Verification items for the finished model (mm, model axes). A direction names the side the tool comes from. Coordinates: 2 decimals unless noted, no trailing zeros. Order: outer loops, then holes, each group sorted by start corner. A loop starts at its lowest first (then second) coordinate and runs counter-clockwise, first axis right, second up. Notation, with made-up numbers: M -13.5,79.25 L 0.5,79.25 A24 ccw 0.5,91.25 Z; hole C 63,69 d6. An arc over 180 degrees is marked long. Return JSON: item names as keys, results as strings.
```python
from build123d import *

# Parameters (mm, degrees)
SKETCH2_W           = 100
SKETCH2_H           = 40
BOSS_EXTRUDE5_DEPTH = 14
SHELL1_T            = -2
SKETCH3_6_R         = 2.5
SKETCH3_6_R_2       = 1.5
CUT_EXTRUDE8_DEPTH  = 56.641710973
CUT_EXTRUDE9_DEPTH  = 12
SKETCH5_W           = 100
SKETCH5_H           = 14
SKETCH5_W_2         = 96
SKETCH5_H_2         = 10
BOSS_EXTRUDE6_DEPTH = 5
SKETCH6_R           = 3
SKETCH6_R_2         = 1.5
SKETCH6_R_3         = 1.58
SKETCH6_R_4         = 1.95
BOSS_EXTRUDE7_DEPTH = 14
SKETCH6_2_R         = 1.5
CUT_EXTRUDE11_DEPTH = 58.628118137
CUT_EXTRUDE12_START = -2
SKETCH6_3_R         = 1.58
SKETCH6_3_R_2       = 1.95
CUT_EXTRUDE12_DEPTH = 56.628118137


with BuildPart() as part:
    # Sketch2 → Boss-Extrude5 (new body)
    with BuildSketch(Plane(origin=(0, 0, 0), x_dir=(1, 0, 0), z_dir=(0, 1, 0))):
        Rectangle(SKETCH2_W, SKETCH2_H)
    extrude(amount=BOSS_EXTRUDE5_DEPTH)

    # Shell1
    shell1_openings = [part.faces().sort_by_distance(p)[0] for p in [
        (0, 7, -20),
        (0, 7, 20),
    ]]
    offset(amount=SHELL1_T, openings=shell1_openings, kind=Kind.INTERSECTION)

    # Sketch3<6> → Cut-Extrude8 (cut, through all)
    with BuildSketch(Plane(origin=(0, 14, 0), x_dir=(1, 0, 0), z_dir=(0, 1, 0))):
        with Locations(Location((-10.944299399, 10.466797681, 0), (0, 0, 270))):
            Circle(SKETCH3_6_R)
        with Locations(Location((-42.214291858, -10, 0), (0, 0, 270))):
            Circle(SKETCH3_6_R_2)
        with Locations(Location((-42.214291858, 10, 0), (0, 0, 270))):
            Circle(SKETCH3_6_R_2)
        with Locations(Location((-22.547984959, 10.466797681, 0), (0, 0, 270))):
            Circle(SKETCH3_6_R_2)
        with Locations(Location((-7.3745, -1.251, 0), (0, 0, 270))):
            Circle(SKETCH3_6_R_2)
        with Locations(Location((7.3745, -1.251, 0), (0, 0, 270))):
            Circle(SKETCH3_6_R_2)
        with Locations(Location((12.650652812, 9.804528549, 0), (0, 0, 270))):
            Circle(SKETCH3_6_R_2)
        with Locations(Location((22.400652812, 9.804528549, 0), (0, 0, 270))):
            Circle(SKETCH3_6_R_2)
        with BuildLine():
            ThreePointArc((7.3745, -15), (14.495799481, -13.012041395), (19.557771218, -7.623040759))
            ThreePointArc((19.557771218, -7.623040759), (18.923772695, -5.598677681), (16.899409617, -6.232676204))
            ThreePointArc((16.899409617, -6.232676204), (12.941948405, -10.445809365), (7.3745, -12))
            ThreePointArc((7.3745, -12), (5.8745, -13.5), (7.3745, -15))
        make_face()
        with BuildLine():
            ThreePointArc((-7.3745, -15), (-14.495799481, -13.012041395), (-19.557771218, -7.623040759))
            ThreePointArc((-19.557771218, -7.623040759), (-18.923772695, -5.598677681), (-16.899409617, -6.232676204))
            ThreePointArc((-16.899409617, -6.232676204), (-12.941948405, -10.445809365), (-7.3745, -12))
            ThreePointArc((-7.3745, -12), (-5.8745, -13.5), (-7.3745, -15))
        make_face()
        with Locations(Location((42.150652812, 10, 0), (0, 0, 270))):
            Circle(SKETCH3_6_R_2)
        with Locations(Location((42.150652812, -10, 0), (0, 0, 270))):
            Circle(SKETCH3_6_R_2)
    extrude(amount=-CUT_EXTRUDE8_DEPTH, mode=Mode.SUBTRACT)

    # Sketch3 → Cut-Extrude9 (cut)
    # profile 1 of 2: a face of its own
    with BuildSketch(Plane(origin=(0, 14, 0), x_dir=(1, 0, 0), z_dir=(0, 1, 0))):
        with BuildLine():
            ThreePointArc((-23.545313619, -9.708587593), (-21.009319529, -1.611135279), (-12.911867215, -4.14712937))
            ThreePointArc((-12.911867215, -4.14712937), (-10.611171791, -6.596461319), (-7.3745, -7.5))
            ThreePointArc((-7.3745, -7.5), (-1.3745, -13.5), (-7.3745, -19.5))
            ThreePointArc((-7.3745, -19.5), (-16.826576095, -16.861389441), (-23.545313619, -9.708587593))
        make_face()
        with BuildLine():
            ThreePointArc((-7.3745, -15), (-14.495799481, -13.012041395), (-19.557771218, -7.623040759))
            ThreePointArc((-19.557771218, -7.623040759), (-18.923772695, -5.598677681), (-16.899409617, -6.232676204))
            ThreePointArc((-16.899409617, -6.232676204), (-12.941948405, -10.445809365), (-7.3745, -12))
            ThreePointArc((-7.3745, -12), (-5.8745, -13.5), (-7.3745, -15))
        make_face(mode=Mode.SUBTRACT)
    # profile 2 of 2: a face of its own
    with BuildSketch(Plane(origin=(0, 14, 0), x_dir=(1, 0, 0), z_dir=(0, 1, 0))):
        with BuildLine():
            ThreePointArc((7.3745, -19.5), (16.826576095, -16.861389441), (23.545313619, -9.708587593))
            ThreePointArc((23.545313619, -9.708587593), (21.009319529, -1.611135279), (12.911867215, -4.14712937))
            ThreePointArc((12.911867215, -4.14712937), (10.611171791, -6.596461319), (7.3745, -7.5))
            ThreePointArc((7.3745, -7.5), (1.3745, -13.5), (7.3745, -19.5))
        make_face()
        with BuildLine():
            ThreePointArc((19.557771218, -7.623040759), (18.923772695, -5.598677681), (16.899409617, -6.232676204))
            ThreePointArc((16.899409617, -6.232676204), (12.941948405, -10.445809365), (7.3745, -12))
            ThreePointArc((7.3745, -12), (5.8745, -13.5), (7.3745, -15))
            ThreePointArc((7.3745, -15), (14.495799481, -13.012041395), (19.557771218, -7.623040759))
        make_face(mode=Mode.SUBTRACT)
    extrude(amount=-CUT_EXTRUDE9_DEPTH, mode=Mode.SUBTRACT)

    # Sketch5 → Boss-Extrude6 (add)
    with BuildSketch(Plane.XY.offset(20)):
        with Locations((0, 7)):
            Rectangle(SKETCH5_W, SKETCH5_H)
        with Locations((0, 7)):
            Rectangle(SKETCH5_W_2, SKETCH5_H_2, mode=Mode.SUBTRACT)
    extrude(amount=BOSS_EXTRUDE6_DEPTH)

    # Sketch6 → Boss-Extrude7 (add, through all)
    # profile 1 of 5: a face of its own
    with BuildSketch(Plane(origin=(0, 14, 0), x_dir=(1, 0, 0), z_dir=(0, 1, 0))):
        with Locations(Location((0, 17, 0), (0, 0, 90))):
            Circle(SKETCH6_R)
        with Locations(Location((0, 17, 0), (0, 0, 270))):
            Circle(SKETCH6_R_2, mode=Mode.SUBTRACT)
    # profile 2 of 5: a face of its own
    with BuildSketch(Plane(origin=(0, 14, 0), x_dir=(1, 0, 0), z_dir=(0, 1, 0))):
        with Locations(Location((0, -22, 0), (0, 0, 270))):
            Circle(SKETCH6_R)
        with Locations(Location((0, -22, 0), (0, 0, 270))):
            Circle(SKETCH6_R_2, mode=Mode.SUBTRACT)
    # profile 3 of 5: a face of its own
    with BuildSketch(Plane(origin=(0, 14, 0), x_dir=(1, 0, 0), z_dir=(0, 1, 0))):
        with Locations(Location((9.804442129, 19.091797681, 0), (0, 0, 144.913560917))):
            Circle(SKETCH6_R_3)
    # profile 4 of 5: a face of its own
    with BuildSketch(Plane(origin=(0, 14, 0), x_dir=(1, 0, 0), z_dir=(0, 1, 0))):
        with Locations(Location((9.804442129, 1.841797681, 0), (0, 0, 270))):
            Circle(SKETCH6_R_3)
    # profile 5 of 5: a face of its own
    with BuildSketch(Plane(origin=(0, 14, 0), x_dir=(1, 0, 0), z_dir=(0, 1, 0))):
        with Locations(Location((-0.944299399, 10.466797681, 0), (0, 0, 270))):
            Circle(SKETCH6_R_4)
    extrude(amount=-BOSS_EXTRUDE7_DEPTH)

    # Sketch6<2> → Cut-Extrude11 (cut, through all)
    with BuildSketch(Plane(origin=(0, 14, 0), x_dir=(1, 0, 0), z_dir=(0, 1, 0))):
        with Locations(Location((0, -22, 0), (0, 0, 270))):
            Circle(SKETCH6_2_R)
        with Locations(Location((0, 17, 0), (0, 0, 270))):
            Circle(SKETCH6_2_R)
    extrude(amount=-CUT_EXTRUDE11_DEPTH, mode=Mode.SUBTRACT)

    # Sketch6<3> → Cut-Extrude12 (cut, through all)
    with BuildSketch(Plane(origin=(0, 14, 0), x_dir=(1, 0, 0), z_dir=(0, 1, 0)).offset(CUT_EXTRUDE12_START)):
        with Locations((9.804442129, 19.091797681)):
            Circle(SKETCH6_3_R)
        with Locations(Location((9.804442129, 1.841797681, 0), (0, 0, 270))):
            Circle(SKETCH6_3_R)
        with Locations(Location((-0.944299399, 10.466797681, 0), (0, 0, 270))):
            Circle(SKETCH6_3_R_2)
    extrude(amount=-CUT_EXTRUDE12_DEPTH, mode=Mode.SUBTRACT)


solid = part.part
```
Q1. Tool access check on faces 1 (the face through (13.012, 1.014, 10.403)), 2 (the face through (0, 7, -14)), 3 (the face through (-48, 7, 2)), 4 (the face through (16.71, 13.01, 16.93)). Record the directions out of +Z, -Z, +X, -X, +Y, -Y that give a thin tool (end or side, any length) a straight path to the whole face; none if there is none.
Values:
{"face 1": "+Y, -Y", "face 2": "none", "face 3": "+Z, -Z", "face 4": "+Y"}
Q2. Cross-section at B-B, the plane y = 4.5. Record the boundary of the cut face in (x, z), and give its area (3 significant figures).
Values:
{"outline": "M -50,-20 L -48,-20 L -48,25 L -50,25 Z; C 0,-17 d6; C 0,22 d6; M 48,-20 L 50,-20 L 50,25 L 48,25 Z; hole C 0,-17 d3; hole C 0,22 d3", "area": "222 mm^2"}
Q3. Cross-section at C-C, the plane z = 13.5. Record the boundary of the cut face in (x, y), and give its area (3 significant figures).
Values:
{"outline": "M -50,0 L -13.62,0 L -13.62,2 L -48,2 L -48,12 L -20.9,12 L -20.9,14 L -50,14 Z; M -5.87,0 L 5.87,0 L 5.87,2 L -5.87,2 Z; M -1.37,12 L 1.37,12 L 1.37,14 L -1.37,14 Z; M 13.62,0 L 50,0 L 50,14 L 20.9,14 L 20.9,12 L 48,12 L 48,2 L 13.62,2 Z", "area": "331 mm^2"}
Q4. Cross-section at D-D, the plane z = -16.5. Record the boundary of the cut face in (x, y).
Values:
{"outline": "M -50,0 L -1.41,0 L -1.41,14 L -50,14 Z; M 1.41,0 L 50,0 L 50,14 L 1.41,14 Z; hole M -48,2 L -2.96,2 L -2.96,12 L -48,12 Z; hole M 2.96,2 L 48,2 L 48,12 L 2.96,12 Z"}
Q5. Draft check along Y on faces 5 (the face through (48, 7, 2)), 6 (the face through (11.186, 13.014, -10.13)). Enter one of: pulls with the +Y half, pulls with the -Y half, needs draft (parallel to the pull), parting line crosses it, or undercut.
Values:
{"face 5": "undercut", "face 6": "needs draft"}
Q6. Material ranges on line 1 along X through (y, z) = (3.25, -17); line 2 along Y through (x, z) = (-22, -3); line 3 along X through (y, z) = (6, -2), recorded low to high.
Values:
{"line 1": "-50 to -48, -3 to -1.5, 1.5 to 3, 48 to 50", "line 2": "0 to 2, 12 to 14", "line 3": "-50 to -48, 48 to 50"}
Q7. Cross-section at A-A, the plane z = 22. Record the boundary of the cut face in (x, y).
Values:
{"outline": "M -50,0 L -1.5,0 L -1.5,14 L -50,14 Z; M 1.5,0 L 50,0 L 50,14 L 1.5,14 Z; hole M -48,2 L -3,2 L -3,12 L -48,12 Z; hole M 3,2 L 48,2 L 48,12 L 3,12 Z"}
